```python
from build123d import *

# Parameters (mm, degrees)
SKIZZE1_W                                            = 20
SKIZZE1_H                                            = 20
AUFSATZ_LINEAR_AUSTRAGEN1_DEPTH                      = 30
STIRNSENKUNG_F_R_M5_ZYLINDERSCHRAUBE_MIT_D           = 5.5
STIRNSENKUNG_F_R_M5_ZYLINDERSCHRAUBE_MIT_CBORE_D     = 10
STIRNSENKUNG_F_R_M5_ZYLINDERSCHRAUBE_MIT_CBORE_DEPTH = 26.9
STIRNSENKUNG_F_R_M4_ZYLINDERSCHRAUBE_MIT_D           = 4.5
STIRNSENKUNG_F_R_M4_ZYLINDERSCHRAUBE_MIT_CBORE_D     = 8
STIRNSENKUNG_F_R_M4_ZYLINDERSCHRAUBE_MIT_CBORE_DEPTH = 27.2
FASE1_SIZE                                           = 3
FASE1_OF_SPIEGELN2_SIZE                              = 3


with BuildPart() as part:
    # Skizze1 → Aufsatz-Linear austragen1 (new body)
    with BuildSketch(Plane(origin=(0, 0, 0), x_dir=(1, 0, 0), z_dir=(0, 1, 0))):
        Polygon((0, -10), (0, -30), (-75, -30), (-75, 30), (-15, 30), (-15, -10), align=None)
        with Locations((-45, 0)):
            Rectangle(SKIZZE1_W, SKIZZE1_H, mode=Mode.SUBTRACT)
    aufsatz_linear_austragen1 = extrude(amount=AUFSATZ_LINEAR_AUSTRAGEN1_DEPTH)

    # Stirnsenkung für M5 Zylinderschraube mit Innensechskant1 (through all)
    with Locations(Plane(origin=(0, 0, 0), x_dir=(-1, 0, 0), z_dir=(0, -1, 0))):
        with Locations((45, 20), (25, 0), (65, 0)):
            stirnsenkung_f_r_m5_zylinderschraube_mit = CounterBoreHole(STIRNSENKUNG_F_R_M5_ZYLINDERSCHRAUBE_MIT_D / 2, STIRNSENKUNG_F_R_M5_ZYLINDERSCHRAUBE_MIT_CBORE_D / 2, STIRNSENKUNG_F_R_M5_ZYLINDERSCHRAUBE_MIT_CBORE_DEPTH)

    # Stirnsenkung für M4 Zylinderschraube mit Innensechskant1 (through all)
    with Locations(Plane(origin=(0, 0, 0), x_dir=(-1, 0, 0), z_dir=(0, -1, 0))):
        with Locations((25, -20), (65, -20)):
            stirnsenkung_f_r_m4_zylinderschraube_mit = CounterBoreHole(STIRNSENKUNG_F_R_M4_ZYLINDERSCHRAUBE_MIT_D / 2, STIRNSENKUNG_F_R_M4_ZYLINDERSCHRAUBE_MIT_CBORE_D / 2, STIRNSENKUNG_F_R_M4_ZYLINDERSCHRAUBE_MIT_CBORE_DEPTH)

    # Fase1
    fase1_edges = [part.edges().sort_by_distance(p)[0] for p in [
        (-75, 15, -30),
        (-15, 15, -30),
        (-15, 15, 10),
        (-75, 15, 30),
    ]]
    chamfer(fase1_edges, length=FASE1_SIZE)

    # Spiegeln2: Aufsatz-Linear austragen1, Stirnsenkung für M5 Zylinderschraube mit Innensechskant1, Stirnsenkung für M4 Zylinderschraube mit Innensechskant1 across plane
    add(aufsatz_linear_austragen1.mirror(Plane(origin=(0, 0, 0), x_dir=(0, 0, 1), z_dir=(1, 0, 0))))
    add(stirnsenkung_f_r_m5_zylinderschraube_mit.mirror(Plane(origin=(0, 0, 0), x_dir=(0, 0, 1), z_dir=(1, 0, 0))), mode=Mode.SUBTRACT)
    add(stirnsenkung_f_r_m4_zylinderschraube_mit.mirror(Plane(origin=(0, 0, 0), x_dir=(0, 0, 1), z_dir=(1, 0, 0))), mode=Mode.SUBTRACT)

    # Fase1 of Spiegeln2
    fase1_of_spiegeln2_edges = [part.edges().sort_by_distance(p)[0] for p in [
        (75, 15, -30),
        (15, 15, -30),
        (15, 15, 10),
        (75, 15, 30),
    ]]
    chamfer(fase1_of_spiegeln2_edges, length=FASE1_OF_SPIEGELN2_SIZE)


solid = part.part
```
Geometry: final body of the model. Coordinates: model frame, mm. A direction names the side the tool comes from. Round coordinates to 2 decimals unless told otherwise and drop trailing zeros. Loops run counter-clockwise (first coordinate to the right, second up) from the corner with the lowest first, then second, coordinate; pieces in that order, holes last. Notation, with made-up numbers: (15.25, 85.25) -> (37.25, 85.25) arc R25 ccw to (37.25, 119.25) -> close; hole circle Ø5 at (88.5, 8). An arc over 180 degrees is marked (long way). Use one line per item in the form item = value.
Item 1: Contact query for flat-ended pins moving along their axis: pin 1 Ø8 at (x, y) = (2.5, 21) entering from -Z; pin 2 Ø7 at (x, z) = (-65, 20) entering from -Y; pin 3 Ø5 at (x, z) = (-44.5, -18.5) entering from -Y. Output: stop coordinate, or through.
Evaluation:
pin_1 = 10
pin_2 = 27.2
pin_3 = 26.9
Item 2: Material intervals for probe 1 along X at (y, z) = (22, -6.5); probe 2 along Z at (x, y) = (65, 9.5); probe 3 along X at (y, z) = (11, 20), sorted ascending.
Evaluation:
probe_1 = -75 to -55, -35 to -15, 15 to 35, 55 to 75
probe_2 = -30 to -5, 5 to 16, 24 to 30
probe_3 = -75 to -69, -61 to -29, -21 to 21, 29 to 61, 69 to 75
Item 3: Access query for faces 1 (the flat face through (-67.2, 26.9, 2.2)), 2 (the flat face through (-73, 15, -29)), 3 (the flat face through (35, 15, 0)). Directions: +Z, -Z, +X, -X, +Y, -Y. A direction counts if a zero-diameter tool reaches every point of the face in a straight line with its end or side. Return the directions, or none.
Evaluation:
face_1 = -Y
face_2 = -Z, -X, +Y, -Y
face_3 = +Y, -Y
Item 4: Cut plane B-B on y = 22.25. Give the number of separate pieces and of enclosed holes in the cut face, then the cut area to 3 significant figures.
Evaluation:
separate_pieces = 1
enclosed_holes = 12
area = 6,310 mm2
Item 5: Draft query along X for faces 4 (the cylindrical face through (27.747, 28.472, -0.121)), 5 (the cylindrical face through (-20, 13, 0)), 6 (the flat face through (-45, 15, -30)), 7 (the flat face through (-74, 15, 28)). Return one class per face: released by +X, released by -X, zero draft, split by the parting line, or undercut.
Evaluation:
face_4 = undercut
face_5 = undercut
face_6 = zero draft
face_7 = released by -X
Item 6: Cut plane D-D on x = -45. Output: boundary loops of the cut face in (y, z), then the cut area to 3 significant figures.
Evaluation:
outline = (0, -30) -> (30, -30) -> (30, -22.75) -> (26.9, -22.75) -> (26.9, -25) -> (0, -25) -> close; (0, -15) -> (26.9, -15) -> (26.9, -17.25) -> (30, -17.25) -> (30, -10) -> (0, -10) -> close; (0, 10) -> (30, 10) -> (30, 30) -> (0, 30) -> close
area = 914 mm2
Item 7: Cut plane A-A on x = -25. Output: boundary loops of the cut face in (y, z).
Evaluation:
outline = (0, -30) -> (30, -30) -> (30, -2.75) -> (26.9, -2.75) -> (26.9, -5) -> (0, -5) -> close; (0, 5) -> (26.9, 5) -> (26.9, 2.75) -> (30, 2.75) -> (30, 17.75) -> (27.2, 17.75) -> (27.2, 16) -> (0, 16) -> close; (0, 24) -> (27.2, 24) -> (27.2, 22.25) -> (30, 22.25) -> (30, 30) -> (0, 30) -> close
